The listing builds one solid part. Answer for the finished solid, in the listing's coordinates (mm). A direction names the side the tool comes from. Round coordinates to 2 decimals unless told otherwise and drop trailing zeros. Order: outer loops, then holes, each group sorted by start corner. A loop starts at its lowest first (then second) coordinate and runs counter-clockwise, first axis right, second up. Notation, with made-up numbers: (-13, -14.5) - (-2, -14.5) arc R21 ccw to (-2, 19.5) - close; hole circle Ø10 at (47, 63.25). An arc over 180 degrees is marked (long way). Write item = value, one per line.
from build123d import *

# Parameters (mm, degrees)
SKETCH067_R          = 22.5
PAD023_DEPTH         = 15
SKETCH073_W          = 45
SKETCH073_H          = 22.5
POCKET041_DEPTH      = 15.001
POCKET041_DEPTH_BACK = 15.001
SKETCH072_W          = 70
SKETCH072_H          = 8
PAD025_DEPTH         = 15
SKETCH069_R          = 20
POCKET042_DEPTH      = 15.001
POCKET042_DEPTH_BACK = 15.001
SKETCH074_R          = 3.25
POCKET043_DEPTH      = 22.501
SKETCH075_R          = 4.75
POCKET047_DEPTH      = 2


with BuildPart() as part:
    # Sketch067 → Pad023 (new body, symmetric)
    with BuildSketch(Plane.XY):
        Circle(SKETCH067_R)
    extrude(amount=PAD023_DEPTH, both=True)

    # Sketch073 → Pocket041 (cut, two sides)
    with BuildSketch(Plane.XY) as pocket041_sk:
        with Locations((0, -11.25)):
            Rectangle(SKETCH073_W, SKETCH073_H)
    extrude(amount=-POCKET041_DEPTH, mode=Mode.SUBTRACT)
    extrude(pocket041_sk.sketch, amount=POCKET041_DEPTH_BACK, mode=Mode.SUBTRACT)

    # Sketch072 → Pad025 (join, symmetric)
    with BuildSketch(Plane.XY):
        with Locations((0, 4)):
            Rectangle(SKETCH072_W, SKETCH072_H)
    extrude(amount=PAD025_DEPTH, both=True)

    # Sketch069 → Pocket042 (cut, two sides)
    with BuildSketch(Plane.XY) as pocket042_sk:
        Circle(SKETCH069_R)
    extrude(amount=-POCKET042_DEPTH, mode=Mode.SUBTRACT)
    extrude(pocket042_sk.sketch, amount=POCKET042_DEPTH_BACK, mode=Mode.SUBTRACT)

    # Sketch074 → Pocket043 (cut, through all)
    with BuildSketch(Plane.XZ):
        with Locations((28, 0)):
            Circle(SKETCH074_R)
        with Locations((-28, 0)):
            Circle(SKETCH074_R)
    extrude(amount=-POCKET043_DEPTH, mode=Mode.SUBTRACT)

    # Sketch075 (on Face13 of Pocket043) → Pocket047 (cut)
    with BuildSketch(Plane(origin=(0, 8, 0), x_dir=(-1, 0, 0), z_dir=(0, 1, 0))):
        with Locations((28, 0)):
            Circle(SKETCH075_R)
        with Locations((-28, 0)):
            Circle(SKETCH075_R)
    extrude(amount=-POCKET047_DEPTH, mode=Mode.SUBTRACT)


with BuildPart() as part_1:
    # Body010 placement: moved
    add(part.part.moved(Location((0, 0, -197.7))))


solid = part_1.part
Q1. Section A-A on x = 28 is taken. Determine the outline of the cut face in (y, z), then the cut area to 3 significant figures.
Model answer:
outline = (0, -212.7) - (8, -212.7) - (8, -202.45) - (6, -202.45) - (6, -200.95) - (0, -200.95) - close; (0, -194.45) - (6, -194.45) - (6, -192.95) - (8, -192.95) - (8, -182.7) - (0, -182.7) - close
area = 182 mm^2
Q2. Section B-B on z = -191.75 is taken. Determine the outline of the cut face in (x, y).
Model answer:
outline = (-35, 0) - (-20, 0) arc R20 cw to (20, 0) - (35, 0) - (35, 8) - (21.03, 8) arc R22.5 ccw to (-21.03, 8) - (-35, 8) - close
Q3. Section D-D on x = -22 is taken. Determine the outline of the cut face in (y, z).
Model answer:
outline = (0, -212.7) - (8, -212.7) - (8, -182.7) - (0, -182.7) - close
Q4. Section C-C on z = -195.75 is taken. Determine the outline of the cut face in (x, y).
Model answer:
outline = (-35, 0) - (-30.6, 0) - (-30.6, 6) - (-32.33, 6) - (-32.33, 8) - (-35, 8) - close; (-25.4, 0) - (-20, 0) arc R20 cw to (20, 0) - (25.4, 0) - (25.4, 6) - (23.67, 6) - (23.67, 8) - (21.03, 8) arc R22.5 ccw to (-21.03, 8) - (-23.67, 8) - (-23.67, 6) - (-25.4, 6) - close; (30.6, 0) - (35, 0) - (35, 8) - (32.33, 8) - (32.33, 6) - (30.6, 6) - close
Q5. Flat-ended cylindrical pins translate along their axes: P1, Ø3, axis at x = 26.5, z = -200, coming from the +Y side; P2, Ø2, axis at x = -9, z = -206, coming from the -Y side; P3, Ø6, axis at x = -28, z = -197.7, coming from the -Y side; P4, Ø11, axis at x = 26, z = -195.5, coming from the +Y side. Find the tip coordinate at first contact, or state that the pin passes through.
Model answer:
P1 = 6
P2 = 17.32
P3 = through
P4 = 9.27
Q6. Determine the mould class of faces 4 (the face through (-33, 8, -197)), 5 (the face through (-35, 4, -197)), 6 (the face through (-32.53, 7.01, -196.27)), 7 (the face through (35, 4, -197)) for opening direction X: released by +X, released by -X, zero draft, split by the parting line, or undercut.
Model answer:
face_4 = zero draft
face_5 = released by -X
face_6 = undercut
face_7 = released by +X
Q7. Find the intervals of material crossed by line 1 (Z direction, x = 28, y = 7.5); line 2 (Z direction, x = -28, y = 3.75); line 3 (Y direction, x = 27.5, z = -188), in increasing order. Write a range as from..to.
Model answer:
line_1 = -212.7..-202.45, -192.95..-182.7
line_2 = -212.7..-200.95, -194.45..-182.7
line_3 = 0..8
Q8. For faces 1 (the face through (23.47, 7.01, -196.27)), 2 (the face through (23, 8, -194)), 3 (the face through (-0.2, 20.5, -212.7)), determine the directions among +Z, -Z, +X, -X, +Y, -Y from which every point of the face is accessible in a straight line to the end or side of a thin tool.
Model answer:
face_1 = +Y
face_2 = +Z, -Z, +X, +Y
face_3 = -Z, +X, -X, +Y, -Y
